Source: CAD feature listing. Evaluate the final solid. Frame: model axes, mm. Coordinates: 2 decimals unless noted, no trailing zeros. Write each loop counter-clockwise with the first axis right and the second up, starting at its lowest first coordinate (ties: lowest second). Pieces come first, ordered by that corner, then holes. Notation, with made-up numbers: M 57.25,10.25 L 100.25,10.25 A13 cw 100.25,23.25 Z; hole C -13.75,72.25 d1. An arc over 180 degrees is marked long. One line per item, written item: value. Start each with the question number.
Item 1: Cut plane C-C, the plane z = 2.45. State how many separate pieces and enclosed holes the cut face has, then the cut area to 3 significant figures.
Item 2: Pin query (flat end, axial travel): P1, Ø1.6, axis at x = -15.5, z = 1.5, coming from the +Y side; P2, Ø6, axis at x = 15.5, y = 54.5, coming from the +Z side; P3, Ø1.5, axis at x = 19, z = 0.5, coming from the -Y side; P4, Ø1, axis at x = -4, z = 2.5, coming from the -Y side. Return the tip coordinate at first contact, or that it passes through.
Item 3: Cut plane D-D, the plane x = -15. Output: boundary loops of the cut face in (y, z), then the cut area to 3 significant figures.
Item 4: Ray query, L1, parallel to X at y = -1, z = 1.85; L2, parallel to X at y = 5, z = 0.1; L3, parallel to Y at x = 23, z = 2.95. Return the intervals inside material, ascending. Write a range as from..to.
Item 5: Cut plane B-B, the plane x = 10.91. Output: boundary loops of the cut face in (y, z), then the cut area to 3 significant figures.
Item 6: Cut plane A-A, the plane y = -1.5. Output: boundary loops of the cut face in (x, z), then the cut area to 3 significant figures.
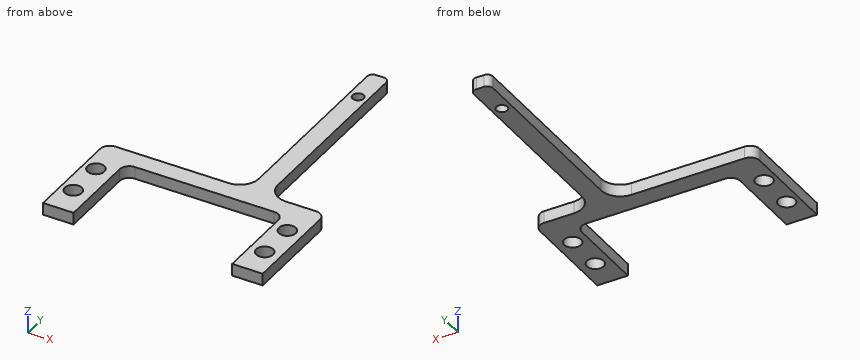
```python
from build123d import *

# Parameters (mm, degrees)
BOSS_EXTRUDE1_DEPTH = 3.18
SKETCH2_R           = 1.47
CUT_EXTRUDE1_DEPTH  = 76.74084037
SKETCH5_W           = 8
SKETCH5_H           = 3.18
BOSS_EXTRUDE2_DEPTH = 3.18
SKETCH6_R           = 2.2225
CUT_EXTRUDE2_DEPTH  = 76.74084037
FILLET1_R           = 5
FILLET2_R           = 1.5
FILLET3_R           = 2.5


with BuildPart() as part:
    # Sketch1 → Boss-Extrude1 (new body)
    with BuildSketch(Plane.XY):
        Polygon((28.75, 15), (13.41, 15), (13.41, 70), (8.41, 70), (8.41, 15), (-28.75, 15), (-28.75, -10), (-20.75, -10), (-20.75, 10), (20.75, 10), (20.75, -10), (28.75, -10), align=None)
    extrude(amount=BOSS_EXTRUDE1_DEPTH)

    # Sketch2 → Cut-Extrude1 (cut, through all)
    with BuildSketch(Plane(origin=(0, 0, 0), x_dir=(-1, 0, 0), z_dir=(0, 0, -1))):
        with Locations((-10.91, 60.25)):
            Circle(SKETCH2_R)
    extrude(amount=-CUT_EXTRUDE1_DEPTH, mode=Mode.SUBTRACT)

    # Sketch5 → Boss-Extrude2 (add)
    with BuildSketch(Plane.XZ.offset(10)):
        with Locations((24.75, 1.59)):
            Rectangle(SKETCH5_W, SKETCH5_H)
        with Locations((-24.75, 1.59)):
            Rectangle(SKETCH5_W, SKETCH5_H)
    extrude(amount=BOSS_EXTRUDE2_DEPTH)

    # Sketch6 → Cut-Extrude2 (cut, through all)
    with BuildSketch(Plane.XY.offset(3.18)):
        with Locations((-25.449, 4.9225)):
            Circle(SKETCH6_R)
        with Locations((-25.449, -5.2375)):
            Circle(SKETCH6_R)
        with Locations((24.649, 4.9225)):
            Circle(SKETCH6_R)
        with Locations((24.649, -5.2375)):
            Circle(SKETCH6_R)
    extrude(amount=-CUT_EXTRUDE2_DEPTH, mode=Mode.SUBTRACT)

    # Fillet1
    fillet1_edges = [part.edges().sort_by_distance(p)[0] for p in [
        (8.41, 15, 1.59),
        (13.41, 15, 1.59),
    ]]
    fillet(fillet1_edges, radius=FILLET1_R)

    # Fillet2
    fillet2_edges = [part.edges().sort_by_distance(p)[0] for p in [
        (8.41, 70, 1.59),
        (13.41, 70, 1.59),
    ]]
    fillet(fillet2_edges, radius=FILLET2_R)

    # Fillet3
    fillet3_edges = [part.edges().sort_by_distance(p)[0] for p in [
        (28.75, 15, 1.59),
        (20.75, 10, 1.59),
        (-20.75, 10, 1.59),
        (-28.75, 15, 1.59),
    ]]
    fillet(fillet3_edges, radius=FILLET3_R)


solid = part.part
```
From the geometry:
1. separate pieces: 1
1. enclosed holes: 5
1. area: 874 mm²
2. P1: stops at y = 15
2. P2: stops at z = 3.18
2. P3: stops at y = 9.5
2. P4: stops at y = 10
3. outline: M 10,0 L 15,0 L 15,3.18 L 10,3.18 Z
3. area: 15.9 mm²
4. L1: x = -28.75..-20.75, 20.75..28.75
4. L2: x = -28.75..-27.67, -23.23..-20.75, 20.75..22.43, 26.87..28.75
4. L3: y = -13.18..-6.73, -3.75..3.43, 6.41..15
5. outline: M 10,0 L 58.78,0 L 58.78,3.18 L 10,3.18 Z; M 61.72,0 L 70,0 L 70,3.18 L 61.72,3.18 Z
5. area: 181 mm²
6. outline: M -28.75,0 L -20.75,0 L -20.75,3.18 L -28.75,3.18 Z; M 20.75,0 L 28.75,0 L 28.75,3.18 L 20.75,3.18 Z
6. area: 50.9 mm²
